from build123d import *

# Parameters (mm, degrees)
BOSS_EXTRUDE1_DEPTH            = 15.875
F_52_0_0635_DIAMETER_HOLE1_D   = 1.6129
SKETCH3_W                      = 7.62
SKETCH3_H                      = 6.985
CUT_EXTRUDE1_DEPTH             = 24.835793107
SKETCH5_R                      = 1.5875
CUT_EXTRUDE2_DEPTH             = 3.302
BOSS_EXTRUDE2_DEPTH            = 1.5875
F_4_40_TAPPED_HOLE1_D          = 2.2606
F_1_16_0_0625_DIAMETER_HOLE1_D = 1.5875


with BuildPart() as part:
    # Sketch1 → Boss-Extrude1 (new body)
    with BuildSketch(Plane(origin=(0, 0, 0), x_dir=(1, 0, 0), z_dir=(0, 1, 0))):
        with BuildLine():
            Line((0, 1.74625), (0, 3.175))
            Line((0, 3.175), (17.49425, 3.175))
            Line((17.49425, 3.175), (17.49425, 0))
            Line((17.49425, 0), (11.43, 0))
            ThreePointArc((11.43, 0), (10.63625, 0.79375), (9.8425, 0))
            Line((9.8425, 0), (1.74625, 0))
            ThreePointArc((1.74625, 0), (0.511464783, 0.511464783), (0, 1.74625))
        make_face()
    extrude(amount=BOSS_EXTRUDE1_DEPTH)

    # #52 (0.0635) Diameter Hole1 (through all)
    with Locations(Plane(origin=(1.74625, 15.875, -1.74625), x_dir=(0, 0, 1), z_dir=(0, 1, 0))):
        with Locations((0, 0)):
            Hole(F_52_0_0635_DIAMETER_HOLE1_D / 2)

    # Sketch3 → Cut-Extrude1 (cut, through all)
    with BuildSketch(Plane(origin=(0, 0, -3.175), x_dir=(-1, 0, 0), z_dir=(0, 0, -1))):
        with Locations((-3.81, 12.3825)):
            Rectangle(SKETCH3_W, SKETCH3_H)
    extrude(amount=-CUT_EXTRUDE1_DEPTH, mode=Mode.SUBTRACT)

    # Sketch5 → Cut-Extrude2 (cut)
    with BuildSketch(Plane.XY):
        with Locations((14.44625, 2.8575)):
            Circle(SKETCH5_R)
    extrude(amount=-CUT_EXTRUDE2_DEPTH, mode=Mode.SUBTRACT)

    # Sketch7 → Boss-Extrude2 (add)
    with BuildSketch(Plane(origin=(0, 0, -3.175), x_dir=(-1, 0, 0), z_dir=(0, 0, -1))):
        Polygon((-17.49425, 0), (0, 0), (0, 8.89), (-7.62, 8.89), (-7.62, 15.875), (-17.49425, 15.875), align=None)
    extrude(amount=BOSS_EXTRUDE2_DEPTH)

    # #4-40 Tapped Hole1 (through all)
    with Locations(Plane(origin=(14.44625, 10.4775, 0), x_dir=(1, 0, 0), z_dir=(0, 0, 1))):
        with Locations((0, 0)):
            Hole(F_4_40_TAPPED_HOLE1_D / 2)

    # 1/16 (0.0625) Diameter Hole1 (through all)
    with Locations(Plane(origin=(14.44625, 2.8575, -3.175), x_dir=(1, 0, 0), z_dir=(0, 0, 1))):
        with Locations((0, 0)):
            Hole(F_1_16_0_0625_DIAMETER_HOLE1_D / 2)


solid = part.part
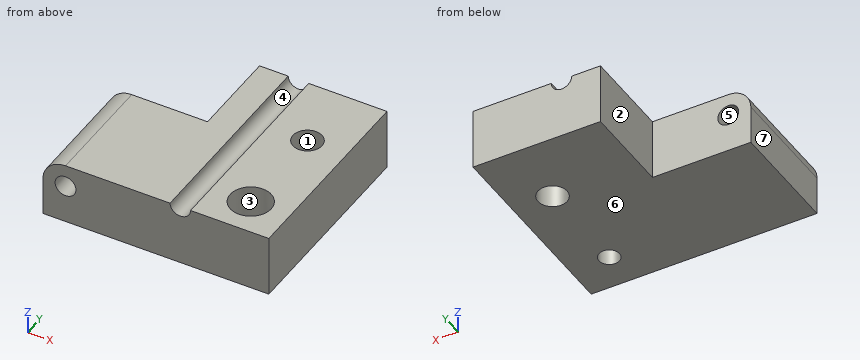
The model under review builds one solid part; all positions refer to its coordinate system, in mm. Face numbers are marked on the shaded views. A direction names the side the tool comes from. Coordinates: 2 decimals unless noted, no trailing zeros. Write each loop counter-clockwise with the first axis right and the second up, starting at its lowest first coordinate (ties: lowest second). Pieces come first, ordered by that corner, then holes. Notation, with made-up numbers: (-9.5, -27.5) - (-3.5, -27.5) arc R12 cw to (-3.5, -23.5) - close; hole circle Ø9 at (-33.5, 62.5). An arc over 180 degrees is marked (long way). Answer as a JSON object with one key per item and string values. Group by question number.
1. Add section D-D (y = 4.25). Give the boundary of the cut face in (x, z) (1 decimal).
2. To check wall thickness, follow probe 1 along X at (y, z) = (10.5, -0.95); probe 2 along Y at (x, z) = (14.75, -1.05) (3 decimals); probe 3 along Z at (x, y) = (2.25, 2.25). State the ranges of each line that lie inside material, in increasing order.
3. Add section B-B (y = 2.5). Give the boundary of the cut face in (x, z) (1 decimal), plus the area to 3 significant figures.
4. Add section A-A (z = -0.6). Give the boundary of the cut face in (x, y) (1 decimal).
5. Mouldability with a two-part tool opening along Z and no side actions: class the marked faces 4, 5, 6 and 7 as pulls with the +Z half, pulls with the -Z half, needs draft (parallel to the pull), parting line crosses it, or undercut.
6. Clearance check with flat-ended pins moving along their axes: pin 1 Ø2 at (x, y) = (14.45, 2.86) entering from +Z (3 decimals); pin 2 Ø1.4 at (y, z) = (13.5, -3) entering from -X. State where each tip first meets the part, or that it passes through.
7. Add section C-C (x = 14.25). Give the boundary of the cut face in (y, z) (1 decimal).
8. Machinability: for the marked faces 1, 2 and 3, which of the approach directions +Z, -Z, +X, -X, +Y, -Y give a long, thin tool a straight path to every point of the face, cutting with its end or side? Answer none if there is none.
Findings:
{
 "1": {"outline": "(0, -4.8) - (17.5, -4.8) - (17.5, 0) - (15.2, 0) - (15.2, -3.2) - (13.7, -3.2) - (13.7, 0) - (11.4, 0) arc R0.8 cw to (9.8, 0) - (1.7, 0) arc R1.7 ccw to (0, -1.7) - close; hole circle Ø1.6 at (1.7, -1.7)"},
 "2": {"probe 1": "7.62 to 13.32, 15.58 to 17.49", "probe 2": "0 to 1.299, 4.416 to 9.389, 11.566 to 15.875", "probe 3": "-4.76 to -2.38, -1.12 to 0"},
 "3": {"outline": "(0, -4.8) - (13.7, -4.8) - (13.7, -3.2) - (12.9, -3.2) - (12.9, 0) - (11.4, 0) arc R0.8 cw to (9.8, 0) - (1.7, 0) arc R1.7 ccw to (0, -1.7) - close; (15.2, -4.8) - (17.5, -4.8) - (17.5, 0) - (16, 0) - (16, -3.2) - (15.2, -3.2) - close; hole circle Ø1.6 at (1.7, -1.7)", "area": "67.6 mm²"},
 "4": {"outline": "(0.4, 0) - (10.1, 0) - (10.1, 15.9) - (7.6, 15.9) - (7.6, 8.9) - (0.4, 8.9) - close; (11.2, 0) - (17.5, 0) - (17.5, 15.9) - (11.2, 15.9) - close; hole circle Ø3.2 at (14.4, 2.9); hole circle Ø2.3 at (14.4, 10.5)"},
 "5": {"face 4": "pulls with the +Z half", "face 5": "undercut", "face 6": "pulls with the -Z half", "face 7": "needs draft"},
 "6": {"pin 1": "z = -3.175", "pin 2": "x = 7.62"},
 "7": {"outline": "(0, -4.8) - (2.1, -4.8) - (2.1, -3.2) - (1.3, -3.2) - (1.3, 0) - (0, 0) - close; (3.6, -4.8) - (9.4, -4.8) - (9.4, 0) - (4.4, 0) - (4.4, -3.2) - (3.6, -3.2) - close; (11.6, -4.8) - (15.9, -4.8) - (15.9, 0) - (11.6, 0) - close"},
 "8": {"face 1": "+Z, -Z", "face 2": "+Z, -Z, -X, +Y", "face 3": "+Z"}
}
